Source: CAD feature listing. Evaluate the final solid. Frame: model axes, mm. Round coordinates to 2 decimals unless told otherwise and drop trailing zeros. Write each loop counter-clockwise with the first axis right and the second up, starting at its lowest first coordinate (ties: lowest second). Pieces come first, ordered by that corner, then holes.
from build123d import *

# Parameters (mm, degrees)
F0_R     = 25.4
F1_DEPTH = 76.2
F1_TAPER = 3
F2_T     = -3.175
F3_R     = 3.175


with BuildPart() as f1:
    # F0 (on Top) → F1 (new body)
    with BuildSketch(Plane.XY):
        Circle(F0_R)
    extrude(amount=F1_DEPTH, taper=F1_TAPER)

    # F2
    f2_openings = [f1.faces().sort_by_distance(p)[0] for p in [
        (0, 0, 76.2),
    ]]
    offset(amount=F2_T, openings=f2_openings)

    # F3
    f3_edges = [f1.edges().sort_by_distance(p)[0] for p in [
        (-22.054248, 0, 3.175),
        (-21.406527, 0, 76.2),
        (-25.4, 0, 0),
    ]]
    fillet(f3_edges, radius=F3_R)


solid = f1.part
1) Section query C-C on z = 51. Return the cut outline in (x, y), then the cut area to 3 significant figures.
Taken from the geometry:
outline: circle Ø45.45 at (0, 0); hole circle Ø39.1 at (0, 0)
area: 422 mm2
2) Contact query for flat-ended pins moving along their axis: P1, Ø5, axis at x = 8, z = 16.5, coming from the -Y side; P2, Ø2, axis at y = 4, z = 65.5, coming from the +X side; P3, Ø4, axis at x = -18, z = 35.5, coming from the -Y side. Output: stop coordinate, or through.
Taken from the geometry:
P1: stops at y = -23.93
P2: stops at x = 21.77
P3: stops at y = -17.27
3) Section query D-D on z = 26. Return the cut outline in (x, y).
Taken from the geometry:
outline: circle Ø48.07 at (0, 0); hole circle Ø41.72 at (0, 0)
4) Material intervals for line 1 (Z direction, x = -6, y = -0.5) (3 decimals); line 2 (Y direction, x = 4, z = 12); line 3 (X direction, y = -3, z = 56), sorted ascending.
Taken from the geometry:
line 1: z = 0 to 3.175
line 2: y = -24.45 to -21.22, 21.22 to 24.45
line 3: x = -22.26 to -19.05, 19.05 to 22.26
5) Pull-direction query (Z, two-part tool) for faces 1 (the face through (0, 0, 0)), 2 (the face through (-18.545, -14.22, 38.755)), 3 (the face through (19.1, 6.02, 41.85)); classes: released by +Z, released by -Z, zero draft, split by the parting line, or undercut.
Taken from the geometry:
face 1: released by -Z
face 2: released by +Z
face 3: undercut
